Here's how the part is built. I have some questions about the finished solid (model axes, mm). A direction names the side the tool comes from. Give positions to 0.01 mm unless a question says otherwise; leave off trailing zeros. Write each loop counter-clockwise with the first axis right and the second up, starting at its lowest first coordinate (ties: lowest second). Pieces come first, ordered by that corner, then holes. Notation, with made-up numbers: M 17.5,14.25 L 55.5,14.25 A30 cw 55.5,50.25 Z; hole C 5,-1.75 d8. An arc over 180 degrees is marked long. Answer as CSV lines item,"result". Start each with the question number.
Q1. On a 3-axis mill with a long thin cutter (end or side, diameter ignored), from which of +Z, -Z, +X, -X, +Y, -Y can I reach the whole of each face in a straight line? I mean faces 5 (the flat face through (56, 53, -59)), 6 (the cylindrical face through (97.87, 64.15, 46.26)), 7 (the cylindrical face through (-38.905, 73.395, -0.224)). Say none if no direction works.
Q2. Suppose I cut it at A-A (z = 112.5). Write out the boundary of the cut face in (x, y), then the cut area to 3 significant figures.
Q3. Thinking about a two-plate mould opening in Z: for faces 1 (the flat face through (15, 0, 0)), 2 (the cylindrical face through (-4.845, 67.311, 69.315)), 3 (the cylindrical face through (-96.99, 64.15, 46.26)), 4 (the cylindrical face through (-68.3, 50.042, -43.545)), which applies, +Z half, -Z half, draft (parallel to the pull), parting line (faces both ways), or undercut?
Q4. If I drill on line 1 along X through (y, z) = (58.25, -56.25); line 2 along Z through (x, y) = (-92.5, 67); line 3 along X through (y, z) = (62.5, 60), over which ranges is the centre line in solid material (lowest first)?
Q5. Suppose I cut it at B-B (x = 3.5). Count the separate pieces of the cut face and the enclosed holes in it, then the cut area to 3 significant figures.
Q6. For pin 1 (12 mm diameter, centred on x = 97.43, z = -56.25, fed in from +Y); pin 2 (6 mm diameter, centred on x = 24, y = 49, fed in from -Z); pin 3 (4 mm diameter, centred on x = -30.5, y = 66, fed in from +Z); pin 4 (8 mm diameter, centred on x = 94, z = -63, fed in from +Y), each with a flat end and sliding along its axis, tell me the tip position at first contact or that it passes through.
```python
from build123d import *

# Parameters (mm, degrees)
SKETCH2_R              = 10
CUT_EXTRUDE1_DEPTH     = 210.076541008
M24_TAPPED_HOLE1_D     = 21
M24_TAPPED_HOLE1_DEPTH = 27
M24_TAPPED_HOLE1_TIP   = 6.3090365
M12_TAPPED_HOLE1_D     = 10.2
M12_TAPPED_HOLE1_DEPTH = 15
M12_TAPPED_HOLE1_TIP   = 3.064389157
SKETCH7_R              = 138
SKETCH7_R_2            = 129
CUT_EXTRUDE2_DEPTH     = 61


with BuildPart() as part:
    # Sketch1 → Revolve1 (revolve)
    with BuildSketch(Plane(origin=(0, 0, 0), x_dir=(0, 0, -1), z_dir=(1, 0, 0))):
        with BuildLine():
            Line((14, 0), (35, 0))
            Line((35, 0), (81, 47))
            Line((81, 47), (81, 53))
            Line((81, 53), (138, 53))
            Line((138, 53), (138, 75))
            Line((138, 75), (93.028360941, 75))
            ThreePointArc((93.028360941, 75), (89.114142828, 76.826684234), (88, 81))
            Line((88, 81), (28, 81))
            Line((28, 81), (28, 35.082903769))
            Line((28, 35.082903769), (14, 27))
            Line((14, 27), (14, 0))
        make_face()
    revolve(axis=Axis((0, 0, 0), (0, 1, 0)))

    # Sketch2 → Cut-Extrude1 (cut, through all)
    with BuildSketch(Plane(origin=(0, 75, 0), x_dir=(1, 0, 0), z_dir=(0, 1, 0))):
        with Locations(Location((0, 112.5, 0), (0, 0, 270))):
            Circle(SKETCH2_R)
        with Locations(Location((97.427857926, 56.25, 0), (0, 0, 270))):
            Circle(SKETCH2_R)
        with Locations(Location((97.427857926, -56.25, 0), (0, 0, 270))):
            Circle(SKETCH2_R)
        with Locations(Location((0, -112.5, 0), (0, 0, 270))):
            Circle(SKETCH2_R)
        with Locations(Location((-97.427857926, -56.25, 0), (0, 0, 270))):
            Circle(SKETCH2_R)
        with Locations(Location((-97.427857926, 56.25, 0), (0, 0, 270))):
            Circle(SKETCH2_R)
    extrude(amount=-CUT_EXTRUDE1_DEPTH, mode=Mode.SUBTRACT)

    # M24 Tapped Hole1
    with Locations(Plane(origin=(0, 81, 0), x_dir=(1, 0, 0), z_dir=(0, 1, 0))):
        with Locations((0, 60), (0, -60)):
            Hole(M24_TAPPED_HOLE1_D / 2, depth=M24_TAPPED_HOLE1_DEPTH)
            with Locations((0, 0, -(M24_TAPPED_HOLE1_DEPTH + M24_TAPPED_HOLE1_TIP / 2))):  # 118° drill point
                Cone(0, M24_TAPPED_HOLE1_D / 2, M24_TAPPED_HOLE1_TIP, mode=Mode.SUBTRACT)

    # M12 Tapped Hole1
    with Locations(Plane(origin=(0, 81, 0), x_dir=(1, 0, 0), z_dir=(0, 1, 0))):
        with Locations((-44, 0), (44, 0)):
            Hole(M12_TAPPED_HOLE1_D / 2, depth=M12_TAPPED_HOLE1_DEPTH)
            with Locations((0, 0, -(M12_TAPPED_HOLE1_DEPTH + M12_TAPPED_HOLE1_TIP / 2))):  # 118° drill point
                Cone(0, M12_TAPPED_HOLE1_D / 2, M12_TAPPED_HOLE1_TIP, mode=Mode.SUBTRACT)

    # Sketch7 → Cut-Extrude2 (cut)
    with BuildSketch(Plane(origin=(0, 81, 0), x_dir=(1, 0, 0), z_dir=(0, 1, 0))):
        Circle(SKETCH7_R)
        with Locations(Location((0, 0, 0), (0, 0, 270))):
            Circle(SKETCH7_R_2, mode=Mode.SUBTRACT)
    extrude(amount=-CUT_EXTRUDE2_DEPTH, mode=Mode.SUBTRACT)


solid = part.part
```
Resolved:
1,face 5,"-Y"
1,face 6,"+Y, -Y"
1,face 7,"+Y"
2,outline,"M -63.12,53 L -10,53 L -10,75 L -63.12,75 Z; M 10,53 L 63.12,53 L 63.12,75 L 10,75 Z"
2,area,"2,340 mm^2"
3,face 1,"draft"
3,face 2,"undercut"
3,face 3,"undercut"
3,face 4,"parting line"
4,line 1,"-116.09 to -107.43, -87.43 to -9.81, 9.81 to 87.43, 107.43 to 116.09"
4,line 2,"-89.92 to -64.95, -47.55 to 47.55, 64.95 to 89.92"
4,line 3,"-114.2 to -106.7, -88.16 to -10.5, 10.5 to 88.16, 106.7 to 114.2"
5,separate pieces,"4"
5,enclosed holes,"0"
5,area,"7,540 mm^2"
6,pin 1,"through"
6,pin 2,"z = -78.23"
6,pin 3,"z = 125.81"
6,pin 4,"y = 75"
